Work out the finished part from the listing and answer in its coordinate system (mm). A direction names the side the tool comes from. Round coordinates to 2 decimals unless told otherwise and drop trailing zeros. Loops run counter-clockwise (first coordinate to the right, second up) from the corner with the lowest first, then second, coordinate; pieces in that order, holes last. Notation, with made-up numbers: M 70,-7 L 107,-7 A13 ccw 107,3 Z; hole C 5.25,12.25 d3. An arc over 180 degrees is marked long. One line per item, written item: value.
```python
from build123d import *

# Parameters (mm, degrees)
F0_W      = 203.2
F0_H      = 76.2
F1_DEPTH  = 50.8
F2_W      = 50.8
F2_H      = 50.8
F3_DEPTH  = 25.4
F4_W      = 203.2
F4_H      = 25.4
F5_DEPTH  = 48.26
F6_W      = 101.6
F6_H      = 25.4
F7_DEPTH  = 25.4
F8_W      = 25.4
F8_H      = 50.8
F9_DEPTH  = 25.4
F11_DEPTH = 50.8


with BuildPart() as f1:
    # F0 (on Front) → F1 (new body)
    with BuildSketch(Plane.XZ):
        with Locations((-101.6, 38.1)):
            Rectangle(F0_W, F0_H)
    extrude(amount=F1_DEPTH)

    # F2 (on face) → F3 (join)
    with BuildSketch(Plane.XY.offset(76.2)):
        with Locations((-177.8, -25.4)):
            Rectangle(F2_W, F2_H)
        with Locations((-25.4, -25.4)):
            Rectangle(F2_W, F2_H)
    extrude(amount=F3_DEPTH)

    # F4 (on face) → F5 (join)
    with BuildSketch(Plane.XZ.offset(50.8)):
        with Locations((-101.6, 12.7)):
            Rectangle(F4_W, F4_H)
    extrude(amount=F5_DEPTH)

    # F6 (on face) → F7 (cut)
    with BuildSketch(Plane.XY.offset(25.4)):
        with Locations((-101.6, -86.36)):
            Rectangle(F6_W, F6_H)
    extrude(amount=-F7_DEPTH, mode=Mode.SUBTRACT)

    # F8 (on face) → F9 (cut)
    with BuildSketch(Plane.XY.offset(101.6)):
        with Locations((-12.7, -25.4)):
            Rectangle(F8_W, F8_H)
        with Locations((-190.5, -25.4)):
            Rectangle(F8_W, F8_H)
    extrude(amount=-F9_DEPTH, mode=Mode.SUBTRACT)

    # F10 (on face) → F11 (join)
    with BuildSketch(Plane.XZ.offset(50.8)):
        Polygon((0, 76.2), (-25.4, 101.6), (-25.4, 76.2), align=None)
        Polygon((-177.8, 101.6), (-203.2, 76.2), (-177.8, 76.2), align=None)
    extrude(amount=-F11_DEPTH)


solid = f1.part
```
1) Find section B-B (y = -16.5). Give the vertices of the cut face in (x, z), then the cut area to 3 significant figures.
Check values:
outline: M -203.2,0 L 0,0 L 0,76.2 L -25.4,101.6 L -50.8,101.6 L -50.8,76.2 L -152.4,76.2 L -152.4,101.6 L -177.8,101.6 L -203.2,76.2 Z
area: 17,400 mm2
2) Find section C-C (z = 6). Give the vertices of the cut face in (x, y).
Check values:
outline: M -203.2,-99.06 L -152.4,-99.06 L -152.4,-73.66 L -50.8,-73.66 L -50.8,-99.06 L 0,-99.06 L 0,0 L -203.2,0 Z
3) Find the intervals of material crossed by probe 1 along X at (y, z) = (-90.5, 7); probe 2 along Z at (x, y) = (-120, -28); probe 3 along Z at (x, y) = (-160.5, -62.5), in increasing order. Write a range as from..to.
Check values:
probe 1: -203.2..-152.4, -50.8..0
probe 2: 0..76.2
probe 3: 0..25.4
4) Find section A-A (z = 80.5). Give the vertices of the cut face in (x, y), then the cut area to 3 significant figures.
Check values:
outline: M -198.9,-50.8 L -152.4,-50.8 L -152.4,0 L -198.9,0 Z; M -50.8,-50.8 L -4.3,-50.8 L -4.3,0 L -50.8,0 Z
area: 4,720 mm2
5) Each of these flat-tipped pins is pushed along its axis until it touches: pin 1 (5 mm diameter, centred on x = -118.5, z = 57, fed in from +Y); pin 2 (2 mm diameter, centred on x = -141, y = -71.5, fed in from +Z); pin 3 (3 mm diameter, centred on x = -85, z = 58, fed in from -Y); pin 4 (10 mm diameter, centred on x = -125.5, y = -36, fed in from +Z). Where does it stop, or does it pass through?
Check values:
pin 1: y = 0
pin 2: z = 25.4
pin 3: y = -50.8
pin 4: z = 76.2
6) For faces 4 (the face through (-203.2, -38, 29)), 5 (the face through (-103, -50.8, 56)), 6 (the face through (-102, -25, 76.2)), 7 (the face through (-152.4, -87, 13)), determine the directions among +Z, -Z, +X, -X, +Y, -Y from which every point of the face is accessible in a straight line to the end or side of a thin tool.
Check values:
face 4: +Z, -Z, -X, +Y, -Y
face 5: +Z, +X, -X, -Y
face 6: +Z, +Y, -Y
face 7: +Z, -Z, -Y
7) Find section D-D (x = -17). Give the vertices of the cut face in (y, z).
Check values:
outline: M -99.06,0 L 0,0 L 0,93.2 L -50.8,93.2 L -50.8,25.4 L -99.06,25.4 Z
8) The mould has two halves that part along X. Classify faces 1 (the face through (-102, -73.66, 13)), 2 (the face through (0, -38, 29)), 3 (the face through (-190.3, -25.8, 89.1)): +X half, -X half, draft (parallel to the pull), parting line (faces both ways), or undercut.
Check values:
face 1: undercut
face 2: +X half
face 3: -X half
